For this review, take the finished solid that the model builds, in its own axes (mm). A direction names the side the tool comes from. Give positions to 0.01 mm unless a question says otherwise; leave off trailing zeros. Order: outer loops, then holes, each group sorted by start corner. A loop starts at its lowest first (then second) coordinate and runs counter-clockwise, first axis right, second up.
from build123d import *

# Parameters (mm, degrees)
BOSS_EXTRUDE1_DEPTH                            = 5.55625
SKETCH2_R                                      = 7.112
CUT_EXTRUDE1_DEPTH                             = 6.55625
CBORE_FOR_4_SOCKET_HEAD_CAP_SCREW1_D           = 3.2639
CBORE_FOR_4_SOCKET_HEAD_CAP_SCREW1_CBORE_D     = 5.55752
CBORE_FOR_4_SOCKET_HEAD_CAP_SCREW1_CBORE_DEPTH = 2.8448
CIRPATTERN1_COUNT                              = 4
FILLET1_R                                      = 5.55625


with BuildPart() as part:
    # Sketch1 → Boss-Extrude1 (new body)
    with BuildSketch(Plane.XY):
        Polygon((0, -16.276714219), (-16.276714219, 0), (0, 16.276714219), (16.276714219, 0), align=None)
    extrude(amount=-BOSS_EXTRUDE1_DEPTH)

    # Sketch2 → Cut-Extrude1 (cut, through all)
    with BuildSketch(Plane.XY):
        Circle(SKETCH2_R)
    extrude(amount=-CUT_EXTRUDE1_DEPTH, mode=Mode.SUBTRACT)

    # CBORE for #4 Socket Head Cap Screw1 (through all)
    with Locations(Plane.XY):
        with Locations((0, 10.668)):
            cbore_for_4_socket_head_cap_screw1 = CounterBoreHole(CBORE_FOR_4_SOCKET_HEAD_CAP_SCREW1_D / 2, CBORE_FOR_4_SOCKET_HEAD_CAP_SCREW1_CBORE_D / 2, CBORE_FOR_4_SOCKET_HEAD_CAP_SCREW1_CBORE_DEPTH)

    # CirPattern1: CBORE for #4 Socket Head Cap Screw1 ×4 about axis
    cirpattern1_axis = Axis((0, 0, 0), (0, 0, 1))
    for i in range(1, CIRPATTERN1_COUNT):
        add(cbore_for_4_socket_head_cap_screw1.rotate(cirpattern1_axis, i * 360 / CIRPATTERN1_COUNT), mode=Mode.SUBTRACT)

    # Fillet1
    fillet1_edges = [part.edges().sort_by_distance(p)[0] for p in [
        (0, -16.276714219, -2.778125),
        (-16.276714219, 0, -2.778125),
        (0, 16.276714219, -2.778125),
        (16.276714219, 0, -2.778125),
    ]]
    fillet(fillet1_edges, radius=FILLET1_R)


solid = part.part
1) Tool access review of faces 5 (the face through (-12.286, 0.212, -4.22)), 6 (the face through (7.955, 0.602, -1.402)): name each direction out of +Z, -Z, +X, -X, +Y, -Y from which nothing blocks a thin tool from reaching the whole face with its end or side.
Answer sheet:
face 5: +Z, -Z
face 6: +Z
2) We need section D-D on z = -2.45. Give the boundary of the cut face in (x, y).
Answer sheet:
outline: (-12.35, -3.93) - (-3.93, -12.35) arc R5.56 ccw to (3.93, -12.35) - (12.35, -3.93) arc R5.56 ccw to (12.35, 3.93) - (3.93, 12.35) arc R5.56 ccw to (-3.93, 12.35) - (-12.35, 3.93) arc R5.56 ccw to start; hole circle Ø5.56 at (-10.67, 0); hole circle Ø14.22 at (0, 0); hole circle Ø5.56 at (0, -10.67); hole circle Ø5.56 at (0, 10.67); hole circle Ø5.56 at (10.67, 0)
3) To check wall thickness, follow line 1 (Y direction, x = 0, z = -3.2); line 2 (X direction, y = -1, z = -3.35); line 3 (Y direction, x = -0.5, z = -0.3). State the ranges of each line that lie inside material, in increasing order.
Answer sheet:
line 1: y = -13.98 to -12.3, -9.04 to -7.11, 7.11 to 9.04, 12.3 to 13.98
line 2: x = -13.88 to -11.96, -9.38 to -7.04, 7.04 to 9.38, 11.96 to 13.88
line 3: y = -13.95 to -13.4, -7.93 to -7.09, 7.09 to 7.93, 13.4 to 13.95
4) We need section C-C on y = -10.25. Give the boundary of the cut face in (x, z).
Answer sheet:
outline: (-6.03, -5.56) - (-1.58, -5.56) - (-1.58, -2.84) - (-2.75, -2.84) - (-2.75, 0) - (-6.03, 0) - close; (1.58, -5.56) - (6.03, -5.56) - (6.03, 0) - (2.75, 0) - (2.75, -2.84) - (1.58, -2.84) - close
5) We need section A-A on y = 0. Give the boundary of the cut face in (x, z).
Answer sheet:
outline: (-13.98, -5.56) - (-12.3, -5.56) - (-12.3, -2.84) - (-13.45, -2.84) - (-13.45, 0) - (-13.98, 0) - close; (-9.04, -5.56) - (-7.11, -5.56) - (-7.11, 0) - (-7.89, 0) - (-7.89, -2.84) - (-9.04, -2.84) - close; (7.11, -5.56) - (9.04, -5.56) - (9.04, -2.84) - (7.89, -2.84) - (7.89, 0) - (7.11, 0) - close; (12.3, -5.56) - (13.98, -5.56) - (13.98, 0) - (13.45, 0) - (13.45, -2.84) - (12.3, -2.84) - close
6) Draft analysis for pull direction X (two halves, no side actions). For faces 1 (the face through (0.212, 12.286, -4.22)), 2 (the face through (13.975, -0.061, -2.817)), 3 (the face through (-0.061, 13.975, -2.817)), 4 (the face through (0.602, -7.955, -1.402)), state which applies: +X half, -X half, draft (parallel to the pull), parting line (faces both ways), or undercut.
Answer sheet:
face 1: undercut
face 2: +X half
face 3: parting line
face 4: undercut
7) Clearance check with flat-ended pins moving along their axes: pin 1 (1.7 mm diameter, centred on x = 9.5, y = -1, fed in from +Z); pin 2 (4.5 mm diameter, centred on x = -1, y = -9.5, fed in from +Z); pin 3 (1 mm diameter, centred on y = 6, z = -1, fed in from -X); pin 4 (2 mm diameter, centred on x = -2.5, z = -3, fed in from +Y). State where each tip first meets the part, or that it passes through.
Answer sheet:
pin 1: stops at z = -2.84
pin 2: stops at z = 0
pin 3: stops at x = -10.78
pin 4: stops at y = 13.77
